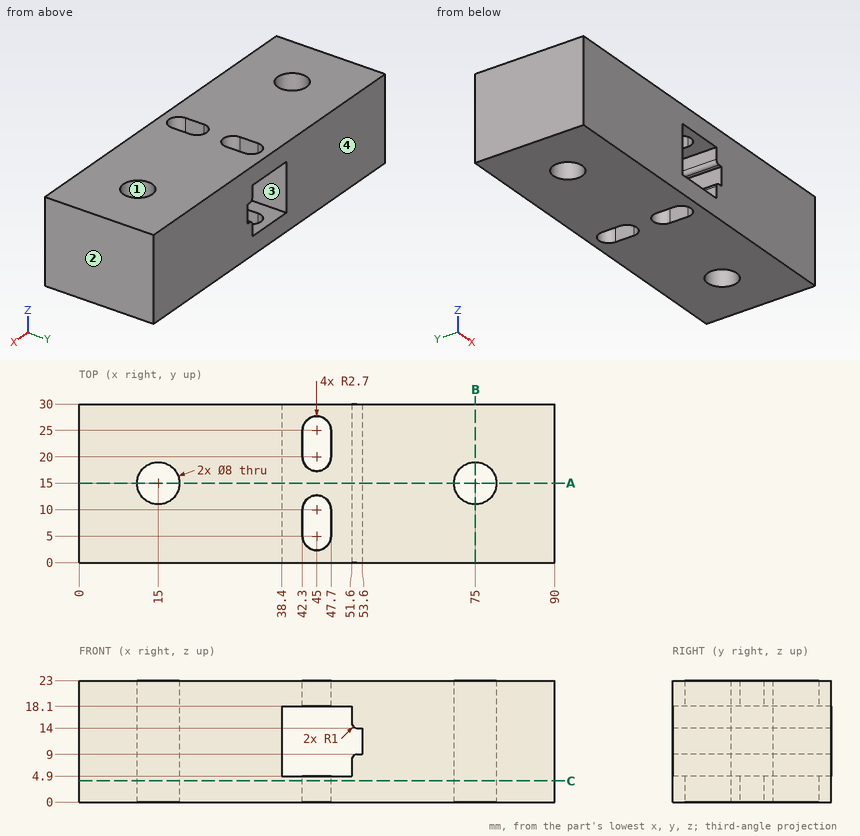
Print and shaded views of the part. All mm, measured from the part's lowest x, y and z. Give positions to 0.01 mm unless a question says otherwise; leave off trailing zeros. Loops run counter-clockwise (first coordinate to the right, second up) from the corner with the lowest first, then second, coordinate; pieces in that order, holes last. Notation, with made-up numbers: (-33.5, -36) -> (22.5, -36) arc R26 cw to (22.5, -15) -> close; hole circle Ø3 at (7, 69.25). An arc over 180 degrees is marked (long way). Use CSV: the item, a comma, the result in double quotes. Start each with the question number.
1) Wall check: line 1 (Z direction, x = 53, y = 25.25); line 2 (Y direction, x = 75, z = 10.5); line 3 (X direction, y = 20.75, z = 7.25). Give the ranges that are in metal, low to high.
2) Slice it at C-C on z = 4. Give the cut face in (x, y).
3) Slice it at B-B on x = 75. Give the cut face in (y, z), plus the area to 3 significant figures.
4) Slice it at A-A on y = 15. Give the cut face in (x, z).
5) Mould opens along X. For the marked faces 1, 2, 3 and 4 say: released by +X, released by -X, zero draft, split by the parting line, or undercut.
Computed values:
1,line 1,"z = 0 to 9, 14 to 23"
1,line 2,"y = 0 to 11, 19 to 30"
1,line 3,"x = 0 to 38.4, 51.6 to 90"
2,outline,"(0, 0) -> (90, 0) -> (90, 30) -> (0, 30) -> close; hole circle Ø8 at (15, 15); hole (42.3, 5) arc R2.7 ccw to (47.7, 5) -> (47.7, 10) arc R2.7 ccw to (42.3, 10) -> close; hole (42.3, 20) arc R2.7 ccw to (47.7, 20) -> (47.7, 25) arc R2.7 ccw to (42.3, 25) -> close; hole circle Ø8 at (75, 15)"
3,outline,"(0, 0) -> (11, 0) -> (11, 23) -> (0, 23) -> close; (19, 0) -> (30, 0) -> (30, 23) -> (19, 23) -> close"
3,area,"506 mm^2"
4,outline,"(0, 0) -> (11, 0) -> (11, 23) -> (0, 23) -> close; (19, 0) -> (71, 0) -> (71, 23) -> (19, 23) -> close; (79, 0) -> (90, 0) -> (90, 23) -> (79, 23) -> close; hole (38.4, 4.9) -> (51.6, 4.9) -> (51.6, 8) arc R1 cw to (52.6, 9) -> (53.6, 9) -> (53.6, 14) -> (52.6, 14) arc R1 cw to (51.6, 15) -> (51.6, 18.1) -> (38.4, 18.1) -> close"
5,face 1,"undercut"
5,face 2,"released by +X"
5,face 3,"undercut"
5,face 4,"zero draft"
